Autodesk Inventor part; units mm, degrees
ref_plane "YZ Plane" through (0, 0, 0) normal (1, 0, 0) x (0, 1, 0)
ref_plane "XZ Plane" through (0, 0, 0) normal (0, 1, 0) x (-1, 0, 0)
ref_plane "XY Plane" through (0, 0, 0) normal (0, 0, 1) x (1, 0, 0)
sketch "Sketch1" plane through (0, 0, 0) normal (0, 1, 0) x (-1, 0, 0)
  line L0 (0, 0) -> (0, 86)
  line L1 (0, 86) -> (-115, 86)
  line L2 (-115, 86) -> (-115, 0)
  line L3 (-115, 0) -> (0, 0)
  dimension "d0" = 86
  dimension "d1" = 115
extrude "Extrusion1" add sketch "Sketch1" along normal blind 2
sketch "Sketch2" plane through (0, 0, 0) normal (0, -1, 0) x (1, 0, 0)
  point P0 (0, 0)
sketch "Sketch3" plane through (0, 0, 0) normal (0, -1, 0) x (1, 0, 0)
  line L0 (112, 83) -> (3, 83)
  line L1 (3, 83) -> (3, 3)
  line L2 (3, 3) -> (112, 3)
  line L3 (112, 3) -> (112, 83)
  line L4 (4, 82) -> (111, 82)
  line L5 (111, 82) -> (111, 4)
  line L6 (111, 4) -> (4, 4)
  line L7 (4, 4) -> (4, 82)
  point P0 (0, 0)
  dimension "d4" = 109
  dimension "d5" = 80
  dimension "d6" = 109
  dimension "d7" = 1
extrude "Extrusion2" add sketch "Sketch3" along normal blind 3
sketch "Sketch4" plane through (0, -3, 0) normal (0, -1, 0) x (1, 0, 0)
  line L0 (2, 84) -> (113, 84)
  line L1 (113, 84) -> (113, 2)
  line L2 (113, 84) -> (195, 84) construction
  line L3 (113, 2) -> (2, 2)
  line L4 (3, 3) -> (112, 3)
  line L5 (2, 2) -> (2, 84)
  line L6 (112, 3) -> (112, 83)
  line L7 (112, 83) -> (3, 83)
  line L8 (3, 83) -> (3, 3)
  line L9 (3, 3) -> (112, 3)
  point P0 (0, 0)
  dimension "d10" = 111
  dimension "d11" = 82
  dimension "d12" = 90
  dimension "d13" = 111
  dimension "d14" = 90
extrude "Extrusion3" add sketch "Sketch4" against normal blind 1
properties part number "cap"
CAD build for the part. Positions are in the model's coordinates, mm. A direction names the side the tool comes from. Round coordinates to 2 decimals unless told otherwise and drop trailing zeros. Write each loop counter-clockwise with the first axis right and the second up, starting at its lowest first coordinate (ties: lowest second). Pieces come first, ordered by that corner, then holes. Notation, with made-up numbers: (70.5, 12) - (113.5, 12) arc R26 cw to (113.5, 29) - close; hole circle Ø1 at (67, 30). An arc over 180 degrees is marked (long way). Write item = value, one per line. Start each with the question number.
Q1. Which spindle directions (+Z, -Z, +X, -X, +Y, -Y) get a long thin tool onto all of the face, cutting with end or side? Do faces 1 (the flat face through (3.8, -3, 43.2)), 2 (the flat face through (4, -1, 42)). Say none if no direction does.
Q2. Mould opens along X. For faces 3 (the flat face through (62, 0, 2)), 4 (the flat face through (58, -1, 4)) say: pulls with the +X half, pulls with the -X half, needs draft (parallel to the pull), parting line crosses it, or undercut.
Q3. Band-saw the part on A-A (z = 57). Give the cut face in (x, y), then the cut area to 3 significant figures.
Q4. Drop flat-ended pins along their axis: pin 1 (6 mm diameter, centred on x = 100.5, z = 66, fed in from -Y); pin 2 (1.1 mm diameter, centred on y = -2.5, z = 63.5, fed in from +X); pin 3 (2.5 mm diameter, centred on y = -1.5, z = 61, fed in from -X). Give the stop position or say it passes through.
Q5. Band-saw the part on B-B (x = 34). Give the cut face in (y, z), then the cut area to 3 significant figures.
Q6. Probe L1, parallel to X at y = -2.1, z = 37.5; L2, parallel to Z at x = 104.5, y = -2.65; L3, parallel to Z at x = 61, y = -0.15. List the from-to ranges inside material, lowest first. Write a range as from..to.
Answers below:
q1.face_1 = +Z, -Z, +X, -X, -Y
q1.face_2 = -Y
q2.face_3 = needs draft
q2.face_4 = undercut
q3.outline = (0, 0) - (3, 0) - (3, -2) - (2, -2) - (2, -3) - (4, -3) - (4, 0) - (111, 0) - (111, -3) - (113, -3) - (113, -2) - (112, -2) - (112, 0) - (115, 0) - (115, 2) - (0, 2) - close
q3.area = 238 mm2
q4.pin_1 = 0
q4.pin_2 = 113
q4.pin_3 = 2
q5.outline = (-3, 2) - (-2, 2) - (-2, 3) - (0, 3) - (0, 0) - (2, 0) - (2, 86) - (0, 86) - (0, 83) - (-2, 83) - (-2, 84) - (-3, 84) - (-3, 82) - (0, 82) - (0, 4) - (-3, 4) - close
q5.area = 180 mm2
q6.L1 = 2..4, 111..113
q6.L2 = 2..4, 82..84
q6.L3 = 3..4, 82..83
